Part print with two shaded views. Sizes in mm from the minimum x, y, z corner. A direction names the side the tool comes from. Coordinates: 2 decimals unless noted, no trailing zeros. Write each loop counter-clockwise with the first axis right and the second up, starting at its lowest first coordinate (ties: lowest second). Pieces come first, ordered by that corner, then holes. Notation, with made-up numbers: (33, 46.25) -> (44, 46.25) arc R29 ccw to (44, 67.25) -> close; hole circle Ø7 at (62, 74.25). An arc over 180 degrees is marked (long way). Write item = value, one per line. Start each with the question number.
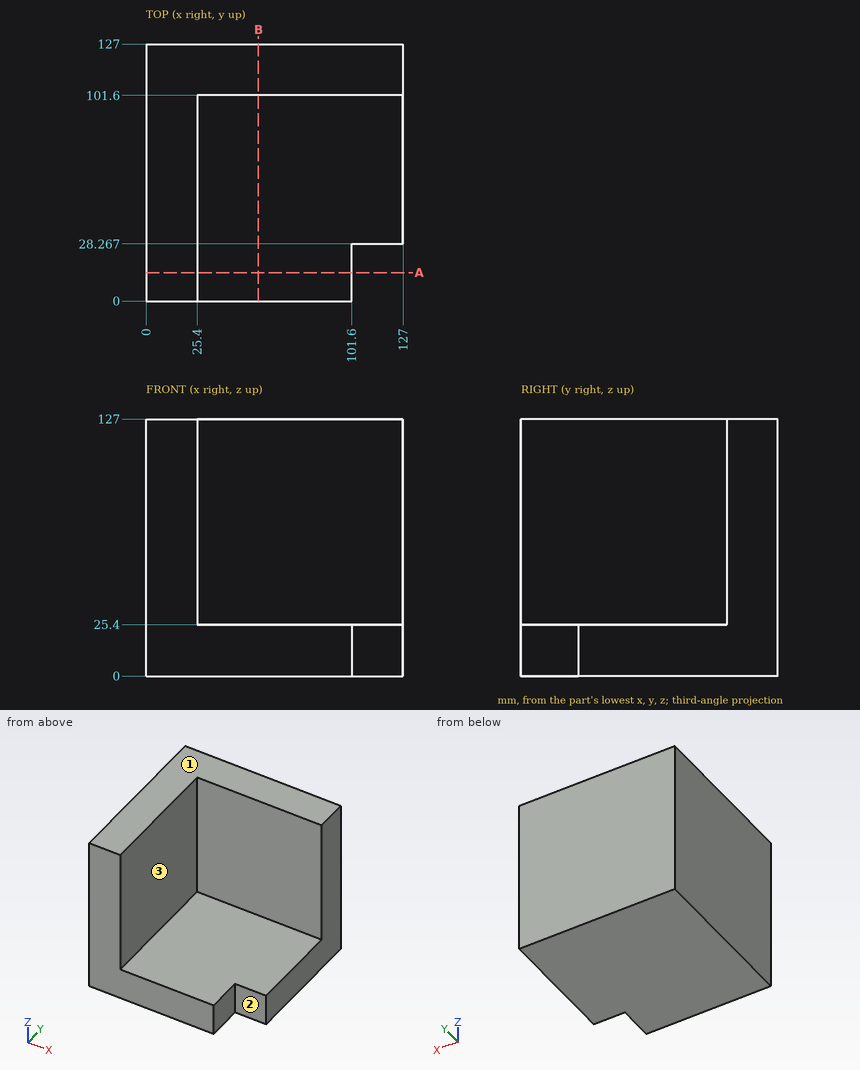
(1) Drop flat-ended pins along their axis: pin 1 Ø20.5 at (x, z) = (120.5, 8) entering from -Y; pin 2 Ø8 at (y, z) = (110.5, 36.5) entering from -X; pin 3 Ø1.5 at (x, z) = (36.5, 42.5) entering from -Y; pin 4 Ø2 at (x, y) = (39, 29) entering from +Z. Give the stop position or say it passes through.
(2) Drill centre lines: line 1 along X through (y, z) = (89, 118.5); line 2 along Y through (x, z) = (118, 87). Where is each one in solid material? Low to high.
(3) 3-axis set-ups, long thin cutter, end or side, ignore diameter. For the marked faces 1, 2 and 3: which of +Z, -Z, +X, -X, +Y, -Y reach the whole face in a straight line?
(4) Saw through at A-A (y = 14). Give the cut face in (x, z).
(5) Saw through at B-B (x = 55.5). Give the cut face in (y, z), then the cut area to 3 significant figures.
Returned:
q1.pin_1 = 28.27
q1.pin_2 = 0
q1.pin_3 = 101.6
q1.pin_4 = 25.4
q2.line_1 = 0 to 25.4
q2.line_2 = 101.6 to 127
q3.face_1 = +Z, +X, -X, +Y, -Y
q3.face_2 = +Z, -Z, +X, -Y
q3.face_3 = +Z, +X, -Y
q4.outline = (0, 0) -> (101.6, 0) -> (101.6, 25.4) -> (25.4, 25.4) -> (25.4, 127) -> (0, 127) -> close
q5.outline = (0, 0) -> (127, 0) -> (127, 127) -> (101.6, 127) -> (101.6, 25.4) -> (0, 25.4) -> close
q5.area = 5,810 mm2
